Work out the finished part from the listing and answer in its coordinate system (mm). Round coordinates to 2 decimals unless told otherwise and drop trailing zeros. Order: outer loops, then holes, each group sorted by start corner. A loop starts at its lowest first (then second) coordinate and runs counter-clockwise, first axis right, second up. Notation, with made-up numbers: M 37,49.25 L 70,49.25 A25 ccw 70,79.25 Z; hole C -23,-19 d8. An arc over 180 degrees is marked long. Answer as a JSON object with one key per item and string values. Group by question number.
from build123d import *

# Parameters (mm, degrees)
F1_DEPTH = 2


with BuildPart() as f1:
    # F0 (on Front) → F1 (new body)
    with BuildSketch(Plane.XZ):
        with BuildLine():
            Line((-13.43, 0), (0, 0))
            Line((0, 0), (0, 39))
            Line((0, 39), (-13.43, 39))
            Line((-13.43, 39), (-13.43, 26.12))
            ThreePointArc((-13.43, 26.12), (-11.626878, 25.373122), (-10.88, 23.57))
            ThreePointArc((-10.88, 23.57), (-11.626878, 21.766878), (-13.43, 21.02))
            Line((-13.43, 21.02), (-13.43, 0))
        make_face()
        with BuildLine():
            Line((-18, 0), (-13.43, 0))
            Line((-13.43, 0), (-13.43, 21.02))
            ThreePointArc((-13.43, 21.02), (-15.233122, 21.766878), (-15.98, 23.57))
            Line((-15.98, 23.57), (-58.02, 23.57))
            ThreePointArc((-58.02, 23.57), (-58.766878, 21.766878), (-60.57, 21.02))
            Line((-60.57, 21.02), (-60.57, 0))
            Line((-60.57, 0), (-56, 0))
            ThreePointArc((-56, 0), (-50.435029, 13.435029), (-37, 19))
            ThreePointArc((-37, 19), (-23.564971, 13.435029), (-18, 0))
        make_face()
        with BuildLine():
            Line((-13.43, 26.12), (-13.43, 39))
            Line((-13.43, 39), (-60.57, 39))
            Line((-60.57, 39), (-60.57, 26.12))
            ThreePointArc((-60.57, 26.12), (-58.766878, 25.373122), (-58.02, 23.57))
            Line((-58.02, 23.57), (-15.98, 23.57))
            ThreePointArc((-15.98, 23.57), (-15.233122, 25.373122), (-13.43, 26.12))
        make_face()
        with BuildLine():
            Line((-60.57, 26.12), (-60.57, 39))
            Line((-60.57, 39), (-74, 39))
            Line((-74, 39), (-74, 0))
            Line((-74, 0), (-60.57, 0))
            Line((-60.57, 0), (-60.57, 21.02))
            ThreePointArc((-60.57, 21.02), (-63.12, 23.57), (-60.57, 26.12))
        make_face()
    extrude(amount=F1_DEPTH)


solid = f1.part
Item 1: Find section C-C (z = 17.5). Give the vertices of the cut face in (x, y), and give its area (3 significant figures).
Item 2: Consider L1, parallel to X at y = -0.7, z = 16.5; L2, parallel to X at y = -0.65, z = 9; L3, parallel to Z at x = -51, y = -1.6. Determine where each line is inside the solid, lowest interval first.
Item 3: Find section A-A (z = 7.5). Give the vertices of the cut face in (x, y), and give its area (3 significant figures).
Item 4: Find section D-D (x = -54). Give the vertices of the cut face in (y, z), and give its area (3 significant figures).
Item 5: Find section B-B (y = -1.55). Give the vertices of the cut face in (x, z).
Responses:
{
 "1": {"outline": "M -74,-2 L -44.4,-2 L -44.4,0 L -74,0 Z; M -29.6,-2 L 0,-2 L 0,0 L -29.6,0 Z", "area": "118 mm^2"},
 "2": {"L1": "x = -74 to -46.42, -27.58 to 0", "L2": "x = -74 to -53.73, -20.27 to 0", "L3": "z = 12.85 to 39"},
 "3": {"outline": "M -74,-2 L -54.46,-2 L -54.46,0 L -74,0 Z; M -19.54,-2 L 0,-2 L 0,0 L -19.54,0 Z", "area": "78.2 mm^2"},
 "4": {"outline": "M -2,8.49 L 0,8.49 L 0,39 L -2,39 Z", "area": "61.0 mm^2"},
 "5": {"outline": "M -74,0 L -56,0 A19 cw -37,19 A19 cw -18,0 L 0,0 L 0,39 L -74,39 Z; hole M -60.57,21.02 A2.55 ccw -58.02,23.57 A2.55 ccw long Z; hole M -15.98,23.57 A2.55 ccw -13.43,21.02 A2.55 ccw -10.88,23.57 A2.55 ccw -13.43,26.12 A2.55 ccw Z"}
}
